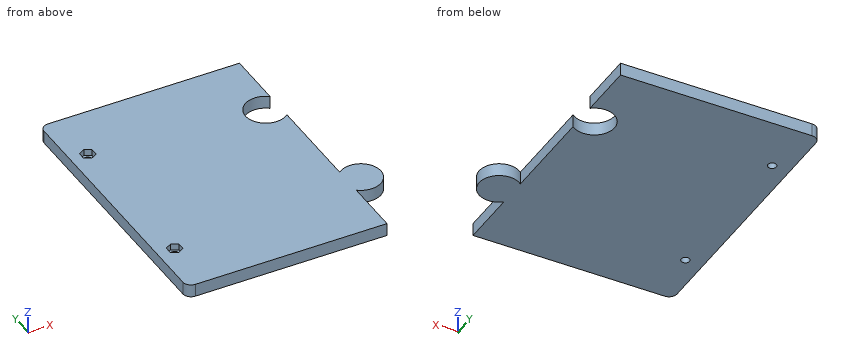
```python
from build123d import *

# Parameters (mm, degrees)
SKETCH_R     = 2.6
PAD_DEPTH    = 8
FILLET_R     = 5
POCKET_DEPTH = 4


with BuildPart() as part:
    # Sketch → Pad (new body)
    with BuildSketch(Plane.XY):
        with BuildLine():
            Line((-62.125, -85), (-62.125, 85))
            Line((-62.125, 85), (62.125, 85))
            Line((62.125, 85), (62.125, 49.669669))
            ThreePointArc((62.125, 49.669669), (41.575, 40), (62.125, 30.330331))
            Line((62.125, 30.330331), (62.125, -30.460477))
            ThreePointArc((62.125, -49.539523), (82.575, -40), (62.125, -30.460477))
            Line((62.125, -49.539523), (62.125, -85))
            Line((62.125, -85), (-62.125, -85))
        make_face()
        with Locations((-51.125, 50)):
            Circle(SKETCH_R, mode=Mode.SUBTRACT)
        with Locations((-51.125, -50)):
            Circle(SKETCH_R, mode=Mode.SUBTRACT)
    extrude(amount=PAD_DEPTH)

    # Fillet
    fillet_edges = [part.edges().sort_by_distance(p)[0] for p in [
        (-62.125, 85, 4),
        (-62.125, -85, 4),
    ]]
    fillet(fillet_edges, radius=FILLET_R)

    # Sketch001 (on Face5 of Fillet) → Pocket (cut)
    with BuildSketch(Plane.XY.offset(8)):
        Polygon((-47.175, 52.280534), (-51.125, 54.561067), (-55.075, 52.280534), (-55.075, 47.719466), (-51.125, 45.438933), (-47.175, 47.719466), align=None)
        Polygon((-47.175, -47.719466), (-51.125, -45.438933), (-55.075, -47.719466), (-55.075, -52.280534), (-51.125, -54.561067), (-47.175, -52.280534), align=None)
    extrude(amount=-POCKET_DEPTH, mode=Mode.SUBTRACT)


solid = part.part
```
Input: part model. Units: mm. Frame: model coordinates. Coordinates: 2 decimals unless noted, no trailing zeros. Loops run counter-clockwise (first coordinate to the right, second up) from the corner with the lowest first, then second, coordinate; pieces in that order, holes last. Notation, with made-up numbers: M 61,14.25 L 102,14.25 A21 ccw 102,37.25 Z; hole C 66,68 d5. An arc over 180 degrees is marked long. One line per item, written item: value.
(1) Section B-B (x = 46). Output: boundary loops of the cut face in (y, z).
Filled in:
outline: M -85,0 L 30.44,0 L 30.44,8 L -85,8 Z; M 49.56,0 L 85,0 L 85,8 L 49.56,8 Z
(2) Line query: line 1 along Y through (x, z) = (54, 0.75); line 2 along X through (y, z) = (-50, 2.9) (3 decimals); line 3 along X through (y, z) = (-61, 2.5) (3 decimals). Output: solid intervals per line, ascending. Write a range as from..to.
Filled in:
line 1: -85..27.45, 52.55..85
line 2: -62.125..-53.725, -48.525..62.125, 62.709..77.541
line 3: -62.125..62.125
(3) Section A-A (z = 6.25). Output: boundary loops of the cut face in (x, y) (3 decimals), and give its area (3 significant figures).
Filled in:
outline: M -62.125,-80 A5 ccw -57.125,-85 L 62.125,-85 L 62.125,-49.54 A12.45 ccw long 62.125,-30.46 L 62.125,30.33 A12.55 cw long 62.125,49.67 L 62.125,85 L -57.125,85 A5 ccw -62.125,80 Z; hole M -55.075,-52.281 L -51.125,-54.561 L -47.175,-52.281 L -47.175,-47.719 L -51.125,-45.439 L -55.075,-47.719 Z; hole M -55.075,47.719 L -51.125,45.439 L -47.175,47.719 L -47.175,52.281 L -51.125,54.561 L -55.075,52.281 Z
area: 21,000 mm^2
(4) Section D-D (x = 70.5). Output: boundary loops of the cut face in (y, z).
Filled in:
outline: M -52.44,0 L -27.56,0 L -27.56,8 L -52.44,8 Z
(5) Pin query (flat end, axial travel): pin 1 (2.5 mm diameter, centred on x = -52.5, y = -50.5, fed in from +Z); pin 2 (4.5 mm diameter, centred on y = -50.5, z = 6, fed in from +X); pin 3 (3 mm diameter, centred on y = 51, z = 6, fed in from +X) (3 decimals). Return the tip coordinate at first contact, or that it passes through.
Filled in:
pin 1: z = 4
pin 2: x = 79.45
pin 3: x = 62.125
(6) Section C-C (y = -23). Output: boundary loops of the cut face in (x, z) (3 decimals).
Filled in:
outline: M -62.125,0 L 62.125,0 L 62.125,8 L -62.125,8 Z
